from build123d import *

# Parameters (mm, degrees)
SKETCH_1_R          = 4
EXTRUDE_1_DEPTH     = 3
SKETCH_3_W          = 15
SKETCH_3_H          = 10
EXTRUDE_3_DEPTH     = 3
SKETCH_2_W          = 3
SKETCH_2_H          = 10
EXTRUDE_4_DEPTH     = 3
SKETCH_4_R          = 1
CUT_EXTRUDE_1_DEPTH = 19.553975315
SKETCH_5_R          = 1.35
CUT_EXTRUDE_2_DEPTH = 19.553975315


with BuildPart() as part:
    # 草图1 → 凸台-拉伸1 (new body)
    with BuildSketch(Plane(origin=(0, 0, 0), x_dir=(1, 0, 0), z_dir=(0, 1, 0))):
        with BuildLine():
            Line((-7.5, 0), (-7.5, 5))
            Line((-7.5, 5), (7.5, 5))
            Line((7.5, 5), (7.5, 0))
            Line((7.5, 0), (7.5, -5))
            ThreePointArc((7.5, -5), (0, -9.013878189), (-7.5, -5))
            Line((-7.5, -5), (-7.5, 0))
        make_face()
        with Locations(Location((0, 0, 0), (0, 0, 270))):
            Circle(SKETCH_1_R, mode=Mode.SUBTRACT)
    extrude(amount=EXTRUDE_1_DEPTH)

    # 草图3 → 凸台-拉伸3 (add)
    with BuildSketch(Plane(origin=(0, 3, 0), x_dir=(1, 0, 0), z_dir=(0, 1, 0))):
        with Locations((0, 10)):
            Rectangle(SKETCH_3_W, SKETCH_3_H)
    extrude(amount=-EXTRUDE_3_DEPTH)

    # 草图2 → 凸台-拉伸4 (add)
    with BuildSketch(Plane(origin=(0, 3, 0), x_dir=(1, 0, 0), z_dir=(0, 1, 0))):
        with Locations((9, 4)):
            Rectangle(SKETCH_2_W, SKETCH_2_H)
        with Locations((-9, 4)):
            Rectangle(SKETCH_2_W, SKETCH_2_H)
    extrude(amount=-EXTRUDE_4_DEPTH)

    # 草图4 → 切除-拉伸1 (cut, through all)
    with BuildSketch(Plane.XZ):
        with Locations((7.5, -10)):
            Circle(SKETCH_4_R)
        with Locations((7.5, 2)):
            Circle(SKETCH_4_R)
        with Locations((-7.5, 2)):
            Circle(SKETCH_4_R)
        with Locations((-7.5, -10)):
            Circle(SKETCH_4_R)
    extrude(amount=-CUT_EXTRUDE_1_DEPTH, mode=Mode.SUBTRACT)

    # 草图5 → 切除-拉伸2 (cut, through all)
    with BuildSketch(Plane.XZ):
        with Locations(Location((0, -12, 0), (0, 0, 270))):
            Circle(SKETCH_5_R)
    extrude(amount=-CUT_EXTRUDE_2_DEPTH, mode=Mode.SUBTRACT)


solid = part.part
Work out the finished part from the listing and answer in its coordinate system (mm). A direction names the side the tool comes from. Round coordinates to 2 decimals unless told otherwise and drop trailing zeros. Loops run counter-clockwise (first coordinate to the right, second up) from the corner with the lowest first, then second, coordinate; pieces in that order, holes last. Notation, with made-up numbers: (68.25, 53.25) -> (76.25, 53.25) arc R17 cw to (76.25, 65.25) -> close; hole circle Ø4 at (24, -8.5). An arc over 180 degrees is marked (long way). Use one line per item in the form item = value.
(1) For a pull along Z with two mould halves and no side action, classify faces 1 (the flat face through (-9, 2, -9)), 2 (the cylindrical face through (0.124, 1.479, 9.013)), 3 (the flat face through (-10.5, 2, -4)), 4 (the cylindrical face through (-3.905, 1.479, -0.867)) as released by +Z, released by -Z, zero draft, split by the parting line, or undercut.
Answer list:
face_1 = released by -Z
face_2 = released by +Z
face_3 = zero draft
face_4 = undercut
(2) Find section A-A on x = 0. Give the vertices of the cut face in (y, z), then the cut area to 3 significant figures.
Answer list:
outline = (0, -15) -> (3, -15) -> (3, -13.35) -> (0, -13.35) -> close; (0, -10.65) -> (3, -10.65) -> (3, -4) -> (0, -4) -> close; (0, 4) -> (3, 4) -> (3, 9.01) -> (0, 9.01) -> close
area = 39.9 mm2
(3) Find section C-C on y = 2.4. Give the vertices of the cut face in (x, z).
Answer list:
outline = (-10.5, -9) -> (-7.5, -9) arc R1 cw to (-7.5, -11) -> (-7.5, -15) -> (7.5, -15) -> (7.5, -11) arc R1 cw to (7.5, -9) -> (10.5, -9) -> (10.5, 1) -> (7.5, 1) arc R1 cw to (7.5, 3) -> (7.5, 5) arc R9.01 ccw to (-7.5, 5) -> (-7.5, 3) arc R1 cw to (-7.5, 1) -> (-10.5, 1) -> close; hole circle Ø8 at (0, 0); hole circle Ø2.7 at (0, -12)
(4) Find section D-D on z = 0. Give the vertices of the cut face in (x, y), then the cut area to 3 significant figures.
Answer list:
outline = (-10.5, 0) -> (-4, 0) -> (-4, 3) -> (-10.5, 3) -> close; (4, 0) -> (10.5, 0) -> (10.5, 3) -> (4, 3) -> close
area = 39.0 mm2
(5) A tool of negligible diameter and unlimited length cuts with its end or side. For faces 5 (the flat face through (-7.5, 2, 4)), 6 (the flat face through (0, 3, -6)), 7 (the flat face through (7.5, 2, 4)), 8 (the flat face through (9, 2, -9)), from which of +Z, -Z, +X, -X, +Y, -Y can it reach the whole face along a straight path? Write none if from no direction.
Answer list:
face_5 = +Z, -X, +Y, -Y
face_6 = +Z, -Z, +X, -X, +Y
face_7 = +Z, +X, +Y, -Y
face_8 = -Z, +X, +Y, -Y
(6) Find section B-B on z = -12. Give the vertices of the cut face in (x, y), then the cut area to 3 significant figures.
Answer list:
outline = (-7.5, 0) -> (-1.35, 0) -> (-1.35, 3) -> (-7.5, 3) -> close; (1.35, 0) -> (7.5, 0) -> (7.5, 3) -> (1.35, 3) -> close
area = 36.9 mm2
(7) Flat-ended cylindrical pins translate along their axes: P1, Ø1, axis at x = -3.5, y = 1.5, coming from the +Z side; P2, Ø1.6, axis at y = 1, z = 4, coming from the -X side; P3, Ø1.6, axis at y = 1.5, z = 4, coming from the +X side. Find the tip coordinate at first contact, or state that the pin passes through.
Answer list:
P1 = 8.5
P2 = -7.5
P3 = 7.5
(8) Straight lines are drawn through the part: line 1 (Z direction, x = -1, y = 2.45); line 2 (X direction, y = 0.95, z = 0); line 3 (Z direction, x = -9.5, y = 1.2). For each, find the intervals that lie inside material, in ascending order.
Answer list:
line_1 = -15 to -12.91, -11.09 to -3.87, 3.87 to 8.96
line_2 = -10.5 to -4, 4 to 10.5
line_3 = -9 to 1
